```python
from build123d import *

# Parameters (mm, degrees)
F2_R           = 2.032
F4_D           = 3.5
F4_CBORE_D     = 6.35
F4_CBORE_DEPTH = 19.685


# Not quite as in the source:
# - a fillet or chamfer that OpenCascade refuses, or shapes differently, is made with other operations: its cross-section is extruded or revolved along the edge and cut away or added


with BuildPart() as f1:
    # F0 (on Right) → F1 (revolve)
    with BuildSketch(Plane.YZ):
        with BuildLine():
            Line((-22.86, 11.0717954744), (-21.59, 10.7315))
            Line((-21.59, 10.7315), (0, 10.7315))
            Line((0, 10.7315), (0, 23.8125))
            Line((0, 23.8125), (-6.35, 23.8125))
            Line((-6.35, 23.8125), (-6.35, 17.0815))
            ThreePointArc((-6.35, 17.0815), (-7.2799359697, 14.8364359697), (-9.525, 13.9065))
            Line((-9.525, 13.9065), (-22.86, 13.9065))
            Line((-22.86, 13.9065), (-22.86, 11.0717954744))
        make_face()
    revolve(axis=Axis((0, -11.43, 0), (0, -1, 0)))

    # F2
    f2_edges = [f1.edges().sort_by_distance(p)[0] for p in [
        (0, -22.86, -13.9065),
    ]]
    fillet(f2_edges, radius=F2_R)

    # F4 (through all)
    with Locations(Plane.XZ.offset(22.86)):
        with Locations((-17.9605122421, 0), (0, 17.9605122421), (17.9605122421, 0), (0, -17.9605122421)):
            CounterBoreHole(F4_D / 2, F4_CBORE_D / 2, F4_CBORE_DEPTH)

    # F5: fillet of radius 3.81 on 1 edges, made by hand

    # F5_s1 → F5_t2 (revolve, cut)
    with BuildSketch(Plane.YZ):
        with BuildLine():
            ThreePointArc((-6.35, 20.0025), (-5.2340768363, 22.6965768363), (-2.54, 23.8125))
            Line((-2.54, 23.8125), (-6.35, 23.8125))
            Line((-6.35, 23.8125), (-6.35, 20.0025))
        make_face()
    revolve(axis=Axis((0, -6.35, 0), (0, -1, 0)), mode=Mode.SUBTRACT)


solid = f1.part
```
Part model, mm, in its own coordinate system. A direction names the side the tool comes from. Round coordinates to 2 decimals unless told otherwise and drop trailing zeros. Order: outer loops, then holes, each group sorted by start corner. A loop starts at its lowest first (then second) coordinate and runs counter-clockwise, first axis right, second up. Notation, with made-up numbers: M 74,6.5 L 83,6.5 A14 ccw 83,17.5 Z; hole C 35.5,64.25 d8. An arc over 180 degrees is marked long. Answer in a Markdown table with one row per item. Add a question column.
Q1. Wall check: L1, parallel to X at y = -5.75, z = -1; L2, parallel to X at y = -5.25, z = 7; L3, parallel to X at y = -20.25, z = 5. Give the ranges that are in metal, low to high. Write a range as from..to.
Q2. Mould opens along Z. For faces 1 (the face through (1.4, -3.175, 16.6)), 2 (the face through (19.3, -3.175, -1.4)), 3 (the face through (8, -22.86, 8)), 4 (the face through (8.462, -15.256, -11.036)) say: +Z half, -Z half, draft (parallel to the pull), parting line (faces both ways), or undercut.
Q3. 3-axis set-ups, long thin cutter, end or side, ignore diameter. For faces 5 (the face through (-13, -6.35, -13)), 6 (the face through (-0.413, -4.821, -14.813)), 7 (the face through (12, -6.35, -13)), 8 (the face through (-13, -6.35, 12)): which of +Z, -Z, +X, -X, +Y, -Y reach the whole face in a straight line?
Q4. Cut at C-C on y = -8. Give the cut face in (x, z), and give its area (3 significant figures).
Q5. Cut at A-A on z = 0. Give the number of separate pieces and of enclosed holes in the cut face, and give its area (3 significant figures).
Q6. Pin check, flat tips, straight feed: pin 1 (5.5 mm diameter, centred on x = -17.96, z = 0, fed in from -Y) (3 decimals); pin 2 (5 mm diameter, centred on x = -18, z = 8, fed in from -Y); pin 3 (10 mm diameter, centred on x = 5.5, y = -17.5, fed in from +Z); pin 4 (3 mm diameter, centred on x = 0, z = 17.96, fed in from -Y). Stop position of each tip, or through.
Established:
| question | item | result |
|---|---|---|
| 1 | L1 | x = -22.03..-20.97, -14.95..-10.68, 10.68..14.95, 20.97..22.03 |
| 1 | L2 | x = -21.57..-8.13, 8.13..21.57 |
| 1 | L3 | x = -12.98..-9.5, 9.5..12.98 |
| 2 | face 1 | undercut |
| 2 | face 2 | undercut |
| 2 | face 3 | draft |
| 2 | face 4 | parting line |
| 3 | face 5 | -Z, -X, -Y |
| 3 | face 6 | -Y |
| 3 | face 7 | -Z, +X, -Y |
| 3 | face 8 | +Z, -X, -Y |
| 4 | outline | C 0,0 d28.59; hole C 0,0 d21.46 |
| 4 | area | 280 mm2 |
| 5 | separate pieces | 4 |
| 5 | enclosed holes | 0 |
| 5 | area | 203 mm2 |
| 6 | pin 1 | stops at y = -3.175 |
| 6 | pin 2 | stops at y = -6.35 |
| 6 | pin 3 | stops at z = 13.9 |
| 6 | pin 4 | passes through |
